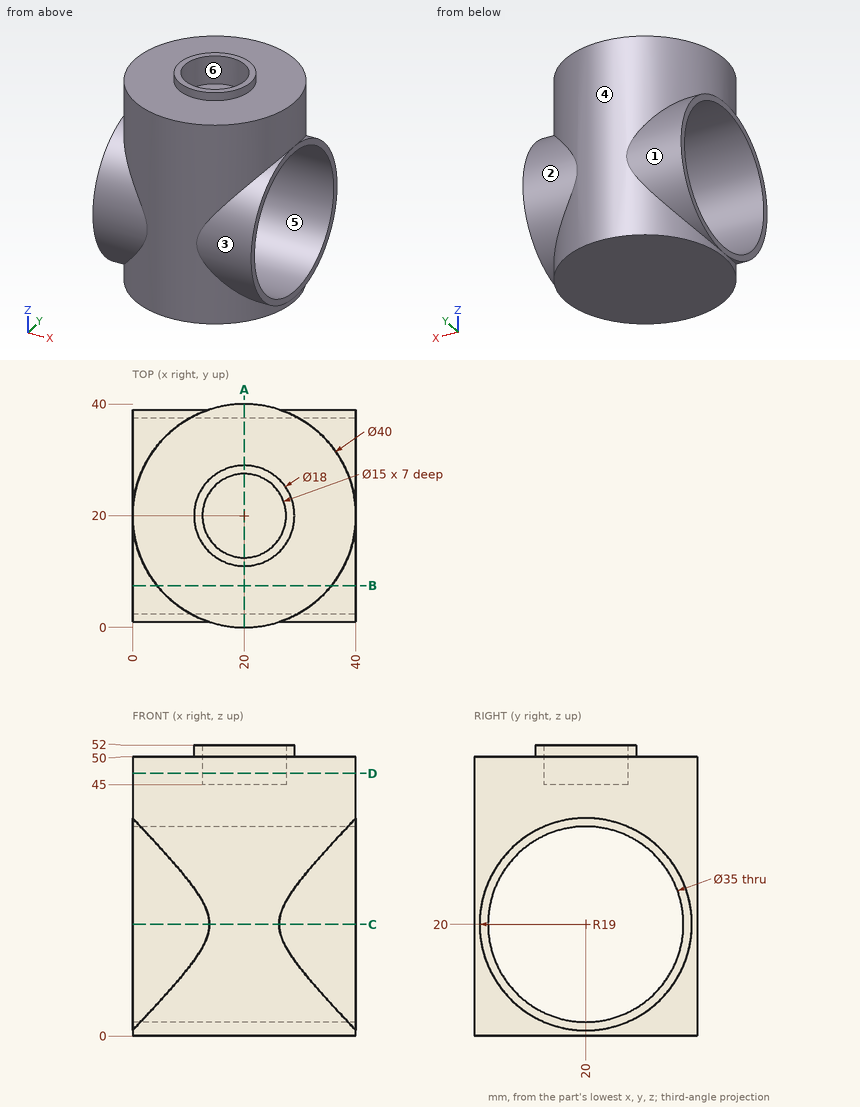
Geometry: see drawing. Coordinates: mm, zero at the bounding-box minimum. A direction names the side the tool comes from. Give positions to 0.01 mm unless a question says otherwise; leave off trailing zeros. Write each loop counter-clockwise with the first axis right and the second up, starting at its lowest first coordinate (ties: lowest second). Pieces come first, ordered by that corner, then holes. Notation, with made-up numbers: M 76.25,84 L 115.25,84 A14 cw 115.25,107 Z; hole C -8.75,-31 d11. An arc over 180 degrees is marked long. Answer in a Markdown table with one row per item. Add a question column.
(1) Ray query, line 1 (Y direction, x = 20, z = 50.25); line 2 (Y direction, x = 20, z = 20); line 3 (Z direction, x = 30.5, y = 22.5). Return the intervals inside material, ascending.
(2) Section C-C on z = 20. Return loops of the section in (x, y) (3 decimals).
(3) Section A-A on x = 20. Return loops of the section in (y, z).
(4) Section D-D on z = 47. Return loops of the section in (x, y).
(5) First-contact query: pin 1 (4 mm diameter, centred on x = 8, z = 43, fed in from +Y); pin 2 (13.5 mm diameter, centred on x = 20, y = 20, fed in from +Z); pin 3 (4 mm diameter, centred on x = 21.5, z = 9.5, fed in from -Y); pin 4 (12 mm diameter, centred on x = 22.5, y = 22.5, fed in from +Z). Flat tips, straight axial feed; report the tip coordinate or a pass-through.
(6) Section B-B on y = 7.5. Return loops of the section in (x, z).
(7) Mould query, pull axis X, two halves, no side actions, for the marked faces 4, 5 and 6. Classes: +X half, -X half, draft (parallel to the pull), parting line (faces both ways), or undercut.
(8) Reachability of the marked faces 1, 2 and 3 from +Z, -Z, +X, -X, +Y, -Y: full face, straight path, thin tool, end or side. Return the list, or none.
Result set:
| question | item | result |
|---|---|---|
| 1 | line 1 | y = 11 to 12.5, 27.5 to 29 |
| 1 | line 2 | y = 0 to 2.5, 37.5 to 40 |
| 1 | line 3 | z = 0 to 2.68, 37.32 to 50 |
| 2 | outline | M 0,1 L 13.755,1 A20 ccw 26.245,1 L 40,1 L 40,2.5 L 0,2.5 Z; M 0,37.5 L 40,37.5 L 40,39 L 26.245,39 A20 ccw 13.755,39 L 0,39 Z |
| 3 | outline | M 0,0 L 40,0 L 40,50 L 29,50 L 29,52 L 27.5,52 L 27.5,45 L 12.5,45 L 12.5,52 L 11,52 L 11,50 L 0,50 Z; hole C 20,20 d35 |
| 4 | outline | C 20,20 d40; hole C 20,20 d15 |
| 5 | pin 1 | stops at y = 37.32 |
| 5 | pin 2 | stops at z = 45 |
| 5 | pin 3 | stops at y = 0 |
| 5 | pin 4 | stops at z = 52 |
| 6 | outline | M 0,5.69 L 4.39,5.69 L 4.39,0 L 35.61,0 L 35.61,5.69 L 40,5.69 L 40,7.75 L 0,7.75 Z; M 0,32.25 L 40,32.25 L 40,34.31 L 35.61,34.31 L 35.61,50 L 4.39,50 L 4.39,34.31 L 0,34.31 Z |
| 7 | face 4 | parting line |
| 7 | face 5 | draft |
| 7 | face 6 | undercut |
| 8 | face 1 | -X, +Y |
| 8 | face 2 | +X, +Y |
| 8 | face 3 | +X, -Y |
